Check sheet for the modelled part. Datum: model origin and axes. Units: mm. Face numbers are marked on the shaded views. A direction names the side the tool comes from. Round coordinates to 2 decimals unless told otherwise and drop trailing zeros. Order: outer loops, then holes, each group sorted by start corner. A loop starts at its lowest first (then second) coordinate and runs counter-clockwise, first axis right, second up. Notation, with made-up numbers: M 63.5,-26 L 119.5,-26 A24 cw 119.5,11 Z; hole C 80,-30.75 d3. An arc over 180 degrees is marked long. One line per item, written item: value. Start each with the question number.
(1) Depth check by flat-ended pin: pin 1 Ø1 at (x, y) = (-33, -1) entering from +Z; pin 2 Ø4 at (x, z) = (-29.5, 8) entering from +Y; pin 3 Ø1.5 at (x, y) = (-32, -1) entering from +Z. Enter the tip coordinate at first touch or a pass-through.
(2) Cross-section at B-B, the plane z = 4. Enter the section's corners in (x, y), and give its area (3 significant figures).
(3) Cross-section at C-C, the plane x = -27.25. Enter the section's corners in (y, z), and give its area (3 significant figures).
(4) Cross-section at A-A, the plane y = -2.5. Enter the section's corners in (x, z).
(5) Cross-section at D-D, the plane y = -9. Enter the section's corners in (x, z), and give its area (3 significant figures).
(6) Thickness scan on L1, parallel to Z at x = -29.75, y = -3.5; L2, parallel to X at y = -2.75, z = 8; L3, parallel to Y at x = -33, z = 7. Record the ranges inside material, lowest first.
(7) Release check for a two-part mould opening along Z. For the marked faces 1, 2 and 3 record: released by +Z, released by -Z, zero draft, split by the parting line, or undercut.
(8) Access from +Z, -Z, +X, -X, +Y, -Y to the whole of each face (thin tool, end or side, straight path). Record for the marked faces 4, 5, 6, 7 and 8.
from build123d import *

# Parameters (mm, degrees)
F0_W         = 8
F0_H         = 10
F0_R         = 3
F1_DEPTH     = 12
F2_W         = 1
F2_H         = 10
F3_DEPTH     = 8
F5_DEPTH     = 9.5
F4_W         = 0.5
F4_H         = 6.5
F6_DEPTH     = 1
F7_R         = 0.5
F8_DEPTH     = 11
F9_R         = 0.5
F10_R        = 0.1
F11_W        = 2
F11_H        = 3
F12_DEPTH    = 0.5
F13_R        = 0.375
F14_DEPTH    = 0.25
F15_W        = 2
F15_H        = 4.5
F16_DEPTH    = 0.5
F17_T1_DEPTH = 6.3301270189


# Not quite as in the source:
# - a fillet or chamfer that OpenCascade refuses, or shapes differently, is made with other operations: its cross-section is extruded or revolved along the edge and cut away or added


with BuildPart() as f1:
    # F0 (on Front) → F1 (new body)
    with BuildSketch(Plane.XZ):
        with Locations((-29.9816446145, 7.3587873485)):
            Rectangle(F0_W, F0_H)
        with Locations((-29.9816446145, 8.3587873485)):
            Circle(F0_R, mode=Mode.SUBTRACT)
    extrude(amount=F1_DEPTH)

    # F2 (on face) → F3 (join, through all)
    with BuildSketch(Plane(origin=(-33.9816446145, 0, 0), x_dir=(0, -1, 0), z_dir=(-1, 0, 0))):
        with Locations((-0.5, 7.3587873485)):
            Rectangle(F2_W, F2_H)
    extrude(amount=-F3_DEPTH)

    # F4 (on face) → F5 (cut)
    with BuildSketch(Plane(origin=(0, 1, 0), x_dir=(-1, 0, 0), z_dir=(0, 1, 0))):
        with BuildLine():
            Line((33.9816446145, 12.3587873485), (29.9816446145, 12.3587873485))
            ThreePointArc((29.9816446145, 12.3587873485), (32.4565183487, 11.3336610826), (33.4816446145, 8.8587873485))
            Line((33.4816446145, 8.8587873485), (33.9816446145, 8.8587873485))
            Line((33.9816446145, 8.8587873485), (33.9816446145, 12.3587873485))
        make_face()
        with BuildLine():
            Line((29.9816446145, 12.3587873485), (25.9816446145, 12.3587873485))
            Line((25.9816446145, 12.3587873485), (25.9816446145, 8.8587873485))
            Line((25.9816446145, 8.8587873485), (26.4816446145, 8.8587873485))
            ThreePointArc((26.4816446145, 8.8587873485), (27.5067708804, 11.3336610826), (29.9816446145, 12.3587873485))
        make_face()
    extrude(amount=-F5_DEPTH, mode=Mode.SUBTRACT)

    # F4 (on face) → F6 (cut)
    with BuildSketch(Plane(origin=(0, 1, 0), x_dir=(-1, 0, 0), z_dir=(0, 1, 0))):
        with Locations((26.2316446145, 5.6087873485)):
            Rectangle(F4_W, F4_H)
        with Locations((33.7316446145, 5.6087873485)):
            Rectangle(F4_W, F4_H)
    extrude(amount=-F6_DEPTH, mode=Mode.SUBTRACT)

    # F7 (on face) → F8 (join)
    with BuildSketch(Plane.XZ):
        with Locations((-29.9816446145, 8.3587873485)):
            Circle(F7_R)
    extrude(amount=F8_DEPTH)

    # F9
    f9_edges = [f1.edges().sort_by_distance(p)[0] for p in [
        (-30.481645, -11, 8.358787),
    ]]
    fillet(f9_edges, radius=F9_R)

    # F10
    f10_edges = [f1.edges().sort_by_distance(p)[0] for p in [
        (-29.981645, -12, 12.358787),
        (-25.981645, -12, 7.358787),
        (-33.981645, -12, 7.358787),
        (-29.981645, -12, 2.358787),
        (-25.981645, -10.25, 12.358787),
        (-33.981645, -10.25, 12.358787),
    ]]
    fillet(f10_edges, radius=F10_R)

    # F11 (on face) → F12 (join)
    with BuildSketch(Plane(origin=(0, 1, 0), x_dir=(-1, 0, 0), z_dir=(0, 1, 0))):
        with Locations((27.4816446145, 3.8587873485)):
            Rectangle(F11_W, F11_H)
        with Locations((32.4816446145, 3.8587873485)):
            Rectangle(F11_W, F11_H)
    extrude(amount=F12_DEPTH)

    # F13 (on face) → F14 (join)
    with BuildSketch(Plane(origin=(0, 1, 0), x_dir=(-1, 0, 0), z_dir=(0, 1, 0))):
        with BuildLine():
            Line((31.4816446145, 6.8587873485), (28.4816446145, 6.8587873485))
            ThreePointArc((28.4816446145, 6.8587873485), (29.9816446145, 6.3587873485), (31.4816446145, 6.8587873485))
        make_face()
        with BuildLine():
            ThreePointArc((31.4816446145, 6.8587873485), (32.217712592, 7.7407533597), (32.4816446145, 8.8587873485))
            ThreePointArc((32.4816446145, 8.8587873485), (28.8636106257, 11.094855326), (28.4816446145, 6.8587873485))
            Line((28.4816446145, 6.8587873485), (31.4816446145, 6.8587873485))
        make_face()
        with BuildLine():
            ThreePointArc((31.4816446145, 6.8587873485), (29.9816446145, 6.3587873485), (28.4816446145, 6.8587873485))
            Line((28.4816446145, 6.8587873485), (28.4816446145, 5.3587873485))
            Line((28.4816446145, 5.3587873485), (28.4816446145, 2.3587873485))
            Line((28.4816446145, 2.3587873485), (31.4816446145, 2.3587873485))
            Line((31.4816446145, 2.3587873485), (31.4816446145, 5.3587873485))
            Line((31.4816446145, 5.3587873485), (31.4816446145, 6.8587873485))
        make_face()
        with Locations((29.9816446145, 4.8587873485)):
            Circle(F13_R, mode=Mode.SUBTRACT)
    extrude(amount=F14_DEPTH)

    # F15 (on face) → F16 (join)
    with BuildSketch(Plane.YZ.offset(-25.9816446145)):
        with Locations((-1, 4.6087873485)):
            Rectangle(F15_W, F15_H)
    extrude(amount=F16_DEPTH)

    # F17: fillet of radius 1 on 1 edges, made by hand

    # F17_s2 → F17_t1 (cut)
    with BuildSketch(Plane.XZ.offset(-2.1650635095)):
        with BuildLine():
            ThreePointArc((-25.9816446145, 6.8587873485), (-25.6156192107, 6.4927619447), (-25.4816446145, 5.9927619447))
            Line((-25.4816446145, 5.9927619447), (-25.4816446145, 6.8587873485))
            Line((-25.4816446145, 6.8587873485), (-25.9816446145, 6.8587873485))
        make_face()
    extrude(amount=F17_T1_DEPTH, mode=Mode.SUBTRACT)


solid = f1.part
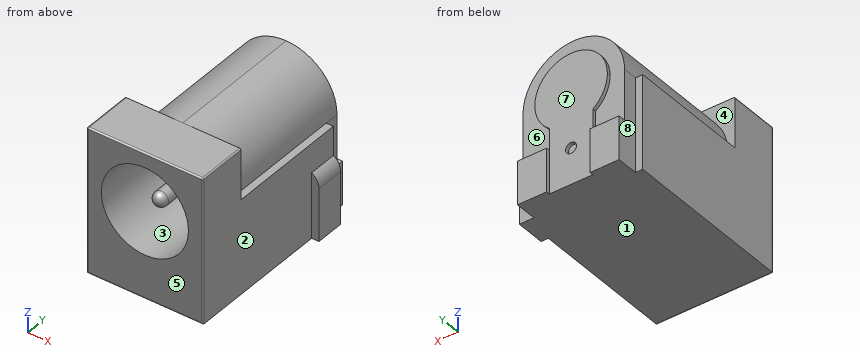
Values found:
1. pin 1: z = 11.29
1. pin 2: y = 1.25
1. pin 3: z = 12.12
2. outline: M -33.98,-11.9 A0.1 ccw -33.88,-12 L -26.08,-12 A0.1 ccw -25.98,-11.9 L -25.98,-2 L -25.48,-2 L -25.48,0 L -26.48,0 L -26.48,1.5 L -28.48,1.5 L -28.48,1.25 L -31.48,1.25 L -31.48,1.5 L -33.48,1.5 L -33.48,0 L -33.98,0 Z
2. area: 107 mm^2
3. outline: M -12,2.46 A0.1 ccw -11.9,2.36 L 1.5,2.36 L 1.5,5.36 L 1,5.36 L 1,11.05 L -8.5,11.05 L -8.5,12.36 L -11.9,12.36 A0.1 ccw -12,12.26 L -12,9.6 L 0,9.6 L 0,7.12 L -12,7.12 Z
3. area: 89.3 mm^2
4. outline: M -33.98,2.36 L -25.98,2.36 L -25.98,8.86 L -26.48,8.86 A3.5 ccw -33.48,8.86 L -33.98,8.86 Z; C -29.98,8.36 d1; hole C -29.98,8.36 d6
5. outline: M -33.98,2.36 L -25.98,2.36 L -25.98,12.26 A0.1 ccw -26.08,12.36 L -33.88,12.36 A0.1 ccw -33.98,12.26 Z; C -29.98,8.36 d1; hole C -29.98,8.36 d6
5. area: 52.5 mm^2
6. L1: 2.36 to 5.37, 7.92 to 8.8, 11.35 to 12.35
6. L2: -33.98 to -32.96, -30.33 to -29.63, -27 to -25.98
6. L3: -12 to 1
7. face 1: released by -Z
7. face 2: zero draft
7. face 3: undercut
8. face 4: +Z, -X, +Y
8. face 5: +Z, -Z, +X, -X, -Y
8. face 6: +Y
8. face 7: +Z, +Y
8. face 8: +Z, -Z, -X, +Y
